Job drawing, mm, ordinate dimensions from the low corner. One solid piece. A direction names the side the tool comes from. Coordinates: 2 decimals unless noted, no trailing zeros. Order: outer loops, then holes, each group sorted by start corner. A loop starts at its lowest first (then second) coordinate and runs counter-clockwise, first axis right, second up. Notation, with made-up numbers: M 87,-29 L 123,-29 A11 cw 123,-24 Z; hole C 71.5,-3.75 d7. An arc over 180 degrees is marked long. Write item = value, one per line. Start each with the question number.
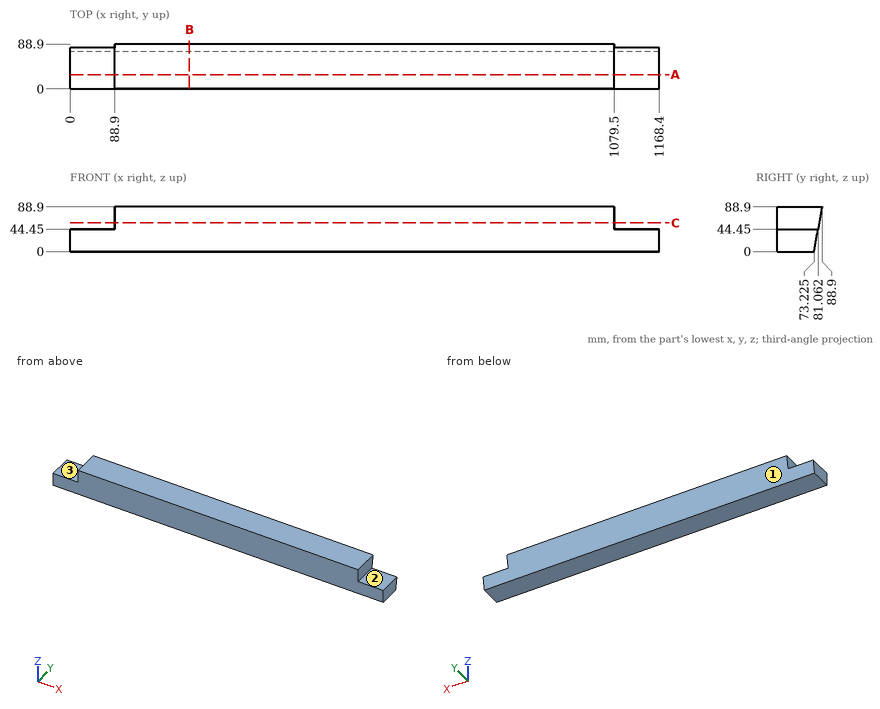
Item 1: Flat gauge pins, fed straight in: pin 1 (1.5 mm diameter, centred on y = 62.5, z = 71.5, fed in from -X); pin 2 (6 mm diameter, centred on x = 387.5, z = 55, fed in from +Y); pin 3 (1 mm diameter, centred on x = 904, z = 45.5, fed in from +Y) (1 decimal). Where does each tip first touch, or does it go through?
Item 2: Wall check: line 1 along X through (y, z) = (83, 57); line 2 along Z through (x, y) = (1082.5, 65); line 3 along Y through (x, z) = (332, 34.5). Give the ranges that are in metal, low to high. Write a range as [from, to].
Item 3: Cut at B-B, the plane x = 236.5. Write the cut outline in (y, z) (1 decimal), and give its area (3 significant figures).
Item 4: Cut at C-C, the plane z = 57. Write the cut outline in (x, y) (1 decimal), and give its area (3 significant figures).
Item 5: 3-axis set-ups, long thin cutter, end or side, ignore diameter. For the marked faces 1, 2 and 3: which of +Z, -Z, +X, -X, +Y, -Y reach the whole face in a straight line?
Item 6: Cut at A-A, the plane y = 28. Write the cut outline in (x, z).
Filled sheet:
q1.pin_1 = 88.9
q1.pin_2 = 83.45
q1.pin_3 = 81.3
q2.line_1 = [88.9, 1079.5]
q2.line_2 = [0, 44.45]
q2.line_3 = [0, 79.31]
q3.outline = M 0,0 L 73.2,0 L 88.9,88.9 L 0,88.9 Z
q3.area = 7,210 mm2
q4.outline = M 88.9,0 L 1079.5,0 L 1079.5,83.3 L 88.9,83.3 Z
q4.area = 82,500 mm2
q5.face_1 = -Z, +X, -X, +Y
q5.face_2 = +Z, +X, +Y, -Y
q5.face_3 = +Z, -X, +Y, -Y
q6.outline = M 0,0 L 1168.4,0 L 1168.4,44.45 L 1079.5,44.45 L 1079.5,88.9 L 88.9,88.9 L 88.9,44.45 L 0,44.45 Z
